Geometry check sheet. Reference: the model listing, model coordinates, mm. A direction names the side the tool comes from. Round coordinates to 2 decimals unless told otherwise and drop trailing zeros. Write each loop counter-clockwise with the first axis right and the second up, starting at its lowest first coordinate (ties: lowest second). Pieces come first, ordered by that corner, then holes. Notation, with made-up numbers: (-4.5, 40) -> (6.5, 40) arc R20 ccw to (6.5, 60) -> close; hole circle Ø3 at (21.25, -20). An arc over 180 degrees is marked (long way). Use a Markdown table: item, result.
```python
from build123d import *

# Parameters (mm, degrees)
F0_W     = 60
F0_H     = 26
F1_DEPTH = 3
F2_W     = 60
F2_H     = 3
F3_DEPTH = 20
F4_W     = 60
F4_H     = 3
F5_DEPTH = 20


with BuildPart() as f1:
    # F0 (on Top) → F1 (new body)
    with BuildSketch(Plane.XY):
        Rectangle(F0_W, F0_H)
        with BuildLine():
            Line((30, -13), (-30, -13))
            Line((-30, -13), (-30, -38))
            Line((-30, -38), (-28.25, -38))
            ThreePointArc((-28.25, -38), (-27.5428932188, -37.7071067812), (-27.25, -37))
            Line((-27.25, -37), (-27.25, -19.5))
            ThreePointArc((-27.25, -19.5), (-26.8106601718, -18.4393398282), (-25.75, -18))
            Line((-25.75, -18), (-24.25, -18))
            ThreePointArc((-24.25, -18), (-23.1893398282, -18.4393398282), (-22.75, -19.5))
            Line((-22.75, -19.5), (-22.75, -37))
            ThreePointArc((-22.75, -37), (-22.4571067812, -37.7071067812), (-21.75, -38))
            Line((-21.75, -38), (-18.75, -38))
            Line((-18.75, -38), (-15.75, -38))
            ThreePointArc((-15.75, -38), (-15.0428932188, -37.7071067812), (-14.75, -37))
            Line((-14.75, -37), (-14.75, -19.5))
            ThreePointArc((-14.75, -19.5), (-14.3106601718, -18.4393398282), (-13.25, -18))
            Line((-13.25, -18), (-11.75, -18))
            ThreePointArc((-11.75, -18), (-10.6893398282, -18.4393398282), (-10.25, -19.5))
            Line((-10.25, -19.5), (-10.25, -37))
            ThreePointArc((-10.25, -37), (-9.9571067812, -37.7071067812), (-9.25, -38))
            Line((-9.25, -38), (-3.25, -38))
            ThreePointArc((-3.25, -38), (-2.5428932188, -37.7071067812), (-2.25, -37))
            Line((-2.25, -37), (-2.25, -19.5))
            ThreePointArc((-2.25, -19.5), (-1.8106601718, -18.4393398282), (-0.75, -18))
            Line((-0.75, -18), (0.75, -18))
            ThreePointArc((0.75, -18), (1.8106601718, -18.4393398282), (2.25, -19.5))
            Line((2.25, -19.5), (2.25, -37))
            ThreePointArc((2.25, -37), (2.5428932188, -37.7071067812), (3.25, -38))
            Line((3.25, -38), (9.25, -38))
            ThreePointArc((9.25, -38), (9.9571067812, -37.7071067812), (10.25, -37))
            Line((10.25, -37), (10.25, -19.5))
            ThreePointArc((10.25, -19.5), (10.6893398282, -18.4393398282), (11.75, -18))
            Line((11.75, -18), (13.25, -18))
            ThreePointArc((13.25, -18), (14.3106601718, -18.4393398282), (14.75, -19.5))
            Line((14.75, -19.5), (14.75, -37))
            ThreePointArc((14.75, -37), (15.0428932188, -37.7071067812), (15.75, -38))
            Line((15.75, -38), (21.75, -38))
            ThreePointArc((21.75, -38), (22.4571067812, -37.7071067812), (22.75, -37))
            Line((22.75, -37), (22.75, -19.5))
            ThreePointArc((22.75, -19.5), (23.1893398282, -18.4393398282), (24.25, -18))
            Line((24.25, -18), (25.75, -18))
            ThreePointArc((25.75, -18), (26.8106601718, -18.4393398282), (27.25, -19.5))
            Line((27.25, -19.5), (27.25, -37))
            ThreePointArc((27.25, -37), (27.5428932188, -37.7071067812), (28.25, -38))
            Line((28.25, -38), (30, -38))
            Line((30, -38), (30, -13))
        make_face()
    extrude(amount=F1_DEPTH)

    # F2 (on face) → F3 (join)
    with BuildSketch(Plane.XY.offset(3)):
        with Locations((0, 11.5)):
            Rectangle(F2_W, F2_H)
    extrude(amount=F3_DEPTH)

    # F4 (on face) → F5 (join)
    with BuildSketch(Plane.XY.offset(3)):
        with Locations((0, -11.5)):
            Rectangle(F4_W, F4_H)
    extrude(amount=F5_DEPTH)


solid = f1.part
```
(1) Section check A-A on z = 19.25. Record the cut outline in (x, y), plus the area to 3 significant figures.
A:
| item | result |
|---|---|
| outline | (-30, -13) -> (30, -13) -> (30, -10) -> (-30, -10) -> close; (-30, 10) -> (30, 10) -> (30, 13) -> (-30, 13) -> close |
| area | 360 mm2 |
(2) Access from +Z, -Z, +X, -X, +Y, -Y to the whole of each face (thin tool, end or side, straight path). Record for faces 3 (the face through (-14.75, -28, 1)), 4 (the face through (0, -10, 13)), 5 (the face through (0, 12, 23)), 6 (the face through (0, -17, 3)), 7 (the face through (-29, -38, 1)).
A:
| item | result |
|---|---|
| face 3 | +Z, -Z, -Y |
| face 4 | +Z, +X, -X |
| face 5 | +Z, +X, -X, +Y, -Y |
| face 6 | +Z, +X, -X, -Y |
| face 7 | +Z, -Z, +X, -X, -Y |
(3) Section check C-C on x = 4. Record the cut outline in (y, z), plus the area to 3 significant figures.
A:
| item | result |
|---|---|
| outline | (-38, 0) -> (13, 0) -> (13, 23) -> (10, 23) -> (10, 3) -> (-10, 3) -> (-10, 23) -> (-13, 23) -> (-13, 3) -> (-38, 3) -> close |
| area | 273 mm2 |
(4) Thickness scan on line 1 (Y direction, x = 24.5, z = 7.5); line 2 (Z direction, x = 20.5, y = -7). Record the ranges inside material, lowest first.
A:
| item | result |
|---|---|
| line 1 | y = -13 to -10, 10 to 13 |
| line 2 | z = 0 to 3 |
(5) Release check for a two-part mould opening along X. For faces 1 (the face through (12, -18, 1)), 2 (the face through (0, -11, 23)) record: +X half, -X half, draft (parallel to the pull), parting line (faces both ways), or undercut.
A:
| item | result |
|---|---|
| face 1 | undercut |
| face 2 | draft |
(6) Section check D-D on y = 1. Record the cut outline in (x, z), plus the area to 3 significant figures.
A:
| item | result |
|---|---|
| outline | (-30, 0) -> (30, 0) -> (30, 3) -> (-30, 3) -> close |
| area | 180 mm2 |
(7) Gauge pin test, flat ends, axial feed: pin 1 Ø20 at (x, y) = (-5, -31.5) entering from +Z; pin 2 Ø1.6 at (x, z) = (12.5, 1) entering from -Y; pin 3 Ø1.5 at (y, z) = (5.5, 5) entering from +X; pin 4 Ø10 at (x, z) = (-1.5, 10.5) entering from -Y. Record the tip position at first contact, or that the pin passes through.
A:
| item | result |
|---|---|
| pin 1 | stops at z = 3 |
| pin 2 | stops at y = -18 |
| pin 3 | passes through |
| pin 4 | stops at y = -13 |
(8) Section check B-B on y = -29.5. Record the cut outline in (x, z), plus the area to 4 significant figures.
A:
| item | result |
|---|---|
| outline | (-30, 0) -> (-27.25, 0) -> (-27.25, 3) -> (-30, 3) -> close; (-22.75, 0) -> (-14.75, 0) -> (-14.75, 3) -> (-22.75, 3) -> close; (-10.25, 0) -> (-2.25, 0) -> (-2.25, 3) -> (-10.25, 3) -> close; (2.25, 0) -> (10.25, 0) -> (10.25, 3) -> (2.25, 3) -> close; (14.75, 0) -> (22.75, 0) -> (22.75, 3) -> (14.75, 3) -> close; (27.25, 0) -> (30, 0) -> (30, 3) -> (27.25, 3) -> close |
| area | 112.5 mm2 |
